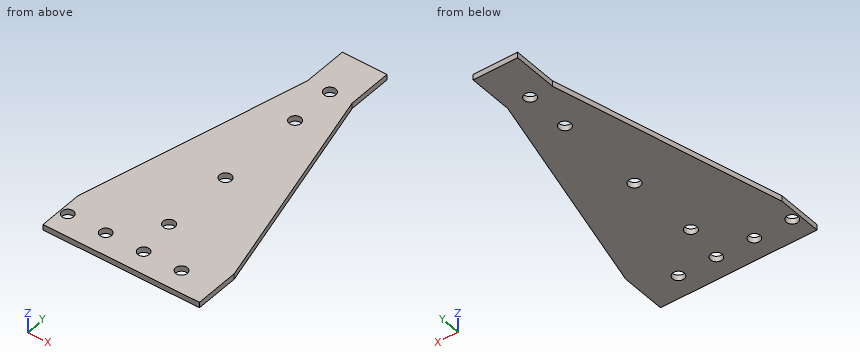
Autodesk Inventor part; units mm, degrees
ref_plane "YZ Plane" through (0, 0, 0) normal (1, 0, 0) x (0, 1, 0)
ref_plane "XZ Plane" through (0, 0, 0) normal (0, 1, 0) x (-1, 0, 0)
ref_plane "XY Plane" through (0, 0, 0) normal (0, 0, 1) x (1, 0, 0)
sketch "Sketch1" plane through (0, 0, 0) normal (0, 0, 1) x (1, 0, 0)
  line L0 (0, 0) -> (-25.4, 0)
  line L1 (-25.4, 0) -> (-25.4, 177.8)
  line L2 (-25.4, 177.8) -> (0, 177.8)
  line L3 (0, 177.8) -> (0, 0)
  line L4 (-25.4, 0) -> (-57.15, 0)
  line L5 (0, 0) -> (31.75, 0)
  line L6 (31.75, 0) -> (31.75, 25.4)
  line L7 (31.75, 25.4) -> (0, 25.4)
  line L8 (-57.15, 0) -> (-57.15, 25.4)
  line L9 (-57.15, 25.4) -> (-25.4, 25.4)
  line L10 (31.75, 25.4) -> (28.575, 25.4)
  line L11 (-25.4, 177.8) -> (-25.4, 152.4)
  line L12 (0, 177.8) -> (0, 150.469)
  line L13 (0, 177.8) -> (0, 152.4)
  line L14 (-57.15, 25.4) -> (-25.4, 152.4)
  line L15 (0, 152.4) -> (31.75, 25.4)
  dimension "d0" = 177.8
  dimension "d3" = 25.4
  dimension "d4" = 31.75
  dimension "d5" = 31.75
  dimension "d6" = 25.4
  dimension "d7" = 3.175
  dimension "d16" = 25.4
extrude "Extrusion1" add sketch "Sketch1" along normal blind 3.175
sketch "Sketch2" plane through (0, 0, 3.175) normal (0, 0, 1) x (1, 0, 0)
  line L0 (0, 177.8) -> (-25.4, 177.8)
  line L1 (-57.15, 25.4) -> (-57.15, 0)
  line L2 (-12.7, 177.8) -> (-12.7, 152.4)
  line L3 (-12.7, 152.4) -> (-12.7, 127)
  circle A0 centre (-12.7, 152.4) radius 3.3782
  circle A1 centre (-12.7, 127) radius 3.3782
  point P0 (0, 0)
  dimension "d10" = 25.4
  dimension "d11" = 25.4
  dimension "d12" = 6.7564
  dimension "d13" = 6.7564
extrude "Extrusion2" cut sketch "Sketch2" against normal blind 25.4
sketch "Sketch4" plane through (0, 0, 3.175) normal (0, 0, 1) x (1, 0, 0)
  circle A0 centre (11.6652, 12.7) radius 3.302
  circle A1 centre (-9.8778, 12.7) radius 3.302
  circle A2 centre (-52.9637, 12.7) radius 3.302
  line L0 (74.422, 18.3438) -> (91.6421, 18.3438)
  circle A3 centre (-31.4207, 12.7) radius 3.302
  point P0 (0, 0)
extrude "Extrusion3" cut sketch "Sketch4" against normal blind 25.4
sketch "Sketch5" plane through (0, 0, 3.175) normal (0, 0, 1) x (1, 0, 0)
  circle A0 centre (-12.7, 127) radius 3.3782
  line L0 (-57.15, 25.4) -> (-57.15, 0)
  line L1 (-12.7, 127) -> (-12.7, 76.2)
  circle A1 centre (-12.7, 76.2) radius 3.3782
  point P0 (0, 0)
  dimension "d22" = 50.8
  dimension "d23" = 6.7564
extrude "Extrusion4" cut sketch "Sketch5" against normal blind 25.4 contours A1
sketch "Sketch6" plane through (0, 0, 3.175) normal (0, 0, 1) x (1, 0, 0)
  circle A0 centre (-12.7, 76.2) radius 3.3782
  line L0 (-57.15, 25.4) -> (-57.15, 0)
  line L1 (-12.7, 76.2) -> (-12.7, 34.925)
  circle A1 centre (-12.7, 34.925) radius 3.3782
  point P0 (0, 0)
  dimension "d26" = 41.275
  dimension "d27" = 6.7564
extrude "Extrusion5" cut sketch "Sketch6" against normal blind 25.4 contours A1
properties part number "winch support" material "Aluminum 6061"
Geometry check sheet. Reference: the model listing, model coordinates, mm. Round coordinates to 2 decimals unless told otherwise and drop trailing zeros. Write each loop counter-clockwise with the first axis right and the second up, starting at its lowest first coordinate (ties: lowest second). Pieces come first, ordered by that corner, then holes.
Item 1: Section check D-D (x = 10.5). Record the boundary of the cut face in (y, z) (3 decimals), plus the area to 3 significant figures.
Determined:
outline: (0, 0) - (9.61, 0) - (9.61, 3.175) - (0, 3.175) - close; (15.79, 0) - (110.4, 0) - (110.4, 3.175) - (15.79, 3.175) - close
area: 331 mm2
Item 2: Section check B-B (y = 12.7). Record the boundary of the cut face in (x, z) (3 decimals), plus the area to 3 significant figures.
Determined:
outline: (-57.15, 0) - (-56.266, 0) - (-56.266, 3.175) - (-57.15, 3.175) - close; (-49.662, 0) - (-34.723, 0) - (-34.723, 3.175) - (-49.662, 3.175) - close; (-28.119, 0) - (-13.18, 0) - (-13.18, 3.175) - (-28.119, 3.175) - close; (-6.576, 0) - (8.363, 0) - (8.363, 3.175) - (-6.576, 3.175) - close; (14.967, 0) - (31.75, 0) - (31.75, 3.175) - (14.967, 3.175) - close
area: 198 mm2
Item 3: Material ranges on line 1 along Y through (x, z) = (-12.7, 2.25); line 2 along Y through (x, z) = (-15, 2.95); line 3 along X through (y, z) = (36.5, 1.55) (3 decimals), recorded low to high.
Determined:
line 1: y = 0 to 10.99, 14.41 to 31.55, 38.3 to 72.82, 79.58 to 123.62, 130.38 to 149.02, 155.78 to 177.8
line 2: y = 0 to 32.45, 37.4 to 73.73, 78.67 to 124.53, 129.47 to 149.93, 154.87 to 177.8
line 3: x = -54.375 to -15.689, -9.711 to 28.975
Item 4: Section check C-C (z = 2). Give the number of separate pieces and of enclosed holes in the cut face, plus the area to 3 significant figures.
Determined:
separate pieces: 1
enclosed holes: 8
area: 9,880 mm2
Item 5: Go/stop test with flat-tipped pins: pin 1 Ø10.5 at (x, y) = (-9.88, 12.7) entering from -Z; pin 2 Ø1 at (y, z) = (171, 1) entering from +X. Record where each tip stops, or that it passes through.
Determined:
pin 1: stops at z = 0
pin 2: stops at x = 0
Item 6: Section check A-A (y = 127). Record the boundary of the cut face in (x, z) (3 decimals).
Determined:
outline: (-31.75, 0) - (-16.078, 0) - (-16.078, 3.175) - (-31.75, 3.175) - close; (-9.322, 0) - (6.35, 0) - (6.35, 3.175) - (-9.322, 3.175) - close
